The listing builds one solid part. Answer for the finished solid, in the listing's coordinates (mm). Face numbers are marked on the shaded views. Coordinates: 2 decimals unless noted, no trailing zeros. Write each loop counter-clockwise with the first axis right and the second up, starting at its lowest first coordinate (ties: lowest second). Pieces come first, ordered by that corner, then holes.
(1) The part is cut by section B-B on x = -2.5. Determine the outline of the cut face in (y, z), plus the area to 3 significant figures.
(2) Given P1, Ø0.6, axis at y = 7.5, z = -0.5, coming from the +X side; P2, Ø6, axis at x = 2, z = 3, coming from the +Y side; P3, Ø0.6, axis at y = 3.5, z = -2, coming from the -X side; P4, Ø5, axis at x = -1, z = -1.5, coming from the +Y side, each flat-ended and moving along its own axis, determine where each tip first touches the part or whether it passes through.
(3) The part is cut by section D-D on x = -0.5. Determine the outline of the cut face in (y, z).
(4) The part is cut by section C-C on z = 2.75. Determine the outline of the cut face in (x, y), plus the area to 3 significant figures.
(5) For a pull along Y with two mould halves and no side action, classify the marked faces 1, 2 and 3 as +Y half, -Y half, draft (parallel to the pull), parting line (faces both ways), or undercut.
(6) Straight lines are drawn through the part: line 1 (Y direction, x = -3.5, z = 0); line 2 (X direction, y = 15.75, z = 0); line 3 (Z direction, x = 0.25, y = 22.5). For each, find the intervals that lie inside material, in ascending order.
(7) The part is cut by section A-A on y = 11. Determine the outline of the cut face in (x, z), plus the area to 3 significant figures.
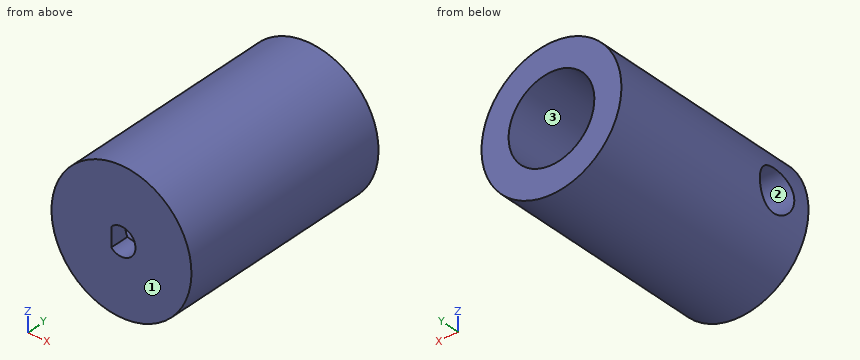
from build123d import *

# Parameters (mm, degrees)
CROQUIS1_R              = 7.75
SALIENTE_EXTRUIR1_DEPTH = 25
VACIADO1_T              = -3
CROQUIS4_R              = 7.75
SALIENTE_EXTRUIR2_DEPTH = 8.7
CORTAR_EXTRUIR1_DEPTH   = 36.6
CROQUIS2_R              = 2.3
CORTAR_EXTRUIR2_DEPTH   = 8.5


with BuildPart() as part:
    # Croquis1 → Saliente-Extruir1 (new body)
    with BuildSketch(Plane(origin=(0, 0, 0), x_dir=(1, 0, 0), z_dir=(0, 1, 0))):
        with Locations(Location((0, 0, 0), (0, 0, 270))):
            Circle(CROQUIS1_R)
    extrude(amount=SALIENTE_EXTRUIR1_DEPTH)

    # Vaciado1
    vaciado1_openings = [part.faces().sort_by_distance(p)[0] for p in [
        (0, 25, 0),
    ]]
    offset(amount=VACIADO1_T, openings=vaciado1_openings, kind=Kind.INTERSECTION)

    # Croquis4 → Saliente-Extruir2 (add)
    with BuildSketch(Plane.XZ):
        with Locations(Location((0, 0, 0), (0, 0, 90))):
            Circle(CROQUIS4_R)
    extrude(amount=-SALIENTE_EXTRUIR2_DEPTH)

    # Croquis3 → Cortar-Extruir1 (cut)
    with BuildSketch(Plane.XZ):
        with BuildLine():
            ThreePointArc((1.55, 0), (0.574750216, 1.439500674), (-1.123757664, 1.067552674))
            Line((-1.123757664, 1.067552674), (-1.123757664, -1.067552674))
            ThreePointArc((-1.123757664, -1.067552674), (0.574750216, -1.439500674), (1.55, 0))
        make_face()
    extrude(amount=-CORTAR_EXTRUIR1_DEPTH, mode=Mode.SUBTRACT)

    # Croquis2 → Cortar-Extruir2 (cut)
    with BuildSketch(Plane(origin=(0, 0, 0), x_dir=(0, 0, -1), z_dir=(1, 0, 0))):
        with Locations((0, 4.19773403)):
            Circle(CROQUIS2_R)
    extrude(amount=-CORTAR_EXTRUIR2_DEPTH, mode=Mode.SUBTRACT)


solid = part.part
Model answer:
1. outline: (0, -7.34) - (25, -7.34) - (25, -4.04) - (8.7, -4.04) - (8.7, 4.04) - (25, 4.04) - (25, 7.34) - (0, 7.34) - close; hole circle Ø4.6 at (4.2, 0)
1. area: 218 mm2
2. P1: stops at x = 7.75
2. P2: stops at y = 25
2. P3: stops at x = -7.47
2. P4: stops at y = 8.7
3. outline: (0, -7.73) - (25, -7.73) - (25, -4.72) - (8.7, -4.72) - (8.7, -1.47) - (5.97, -1.47) arc R2.3 cw to (2.43, -1.47) - (0, -1.47) - close; (0, 1.47) - (2.43, 1.47) arc R2.3 cw to (5.97, 1.47) - (8.7, 1.47) - (8.7, 4.72) - (25, 4.72) - (25, 7.73) - (0, 7.73) - close
4. outline: (-7.25, 0) - (7.25, 0) - (7.25, 25) - (3.87, 25) - (3.87, 8.7) - (-3.87, 8.7) - (-3.87, 25) - (-7.25, 25) - close
4. area: 236 mm2
5. face 1: -Y half
5. face 2: undercut
5. face 3: draft
6. line 1: y = 0 to 1.9, 6.5 to 8.7
6. line 2: x = -7.75 to -4.75, 4.75 to 7.75
6. line 3: z = -7.75 to -4.74, 4.74 to 7.75
7. outline: circle Ø15.5 at (0, 0); hole circle Ø9.5 at (0, 0)
7. area: 118 mm2
